Autodesk Inventor part; units mm, degrees
ref_plane "YZ Plane" through (0, 0, 0) normal (1, 0, 0) x (0, 1, 0)
ref_plane "XZ Plane" through (0, 0, 0) normal (0, 1, 0) x (-1, 0, 0)
ref_plane "XY Plane" through (0, 0, 0) normal (0, 0, 1) x (1, 0, 0)
sketch "スケッチ1" plane through (0, 0, 0) normal (0, 0, 1) x (1, 0, 0)
  line L0 (-75, -5) -> (-75, 5)
  line L1 (-75, 5) -> (10, 5)
  line L2 (10, 5) -> (10, -41.5)
  line L3 (10, -41.5) -> (0, -41.5)
  line L4 (0, -41.5) -> (0, -5)
  line L5 (0, -5) -> (-75, -5)
  point P0 (0, 0)
  dimension "d0" = 85
  dimension "d1" = 46.5
  dimension "d2" = 10
  dimension "d3" = 10
  dimension "d4" = 10
  dimension "d6" = 5
extrude "押し出し1" add sketch "スケッチ1" along normal blind 5 and the other way blind 5
sketch "スケッチ2" plane through (0, -41.5, 5) normal (0, -1, 0) x (1, 0, 0)
  circle A0 centre (5, -5) radius 7.5
  line L0 (0, -10) -> (0, 0)
  point P0 (0, -5)
  point P1 (0, -5)
  dimension "d11" = 15
  dimension "d12" = 5
  dimension "d13" = 5
extrude "押し出し2" add sketch "スケッチ2" against normal blind 20
sketch "スケッチ3" plane through (-75, -5, 5) normal (-1, 0, 0) x (0, 0, 1)
  circle A0 centre (-5, 5) radius 7.5
  dimension "d16" = 15
extrude "押し出し3" add sketch "スケッチ3" against normal blind 20
properties part number "r_link_wr2wp"
Could you check a few things on this model? Use its own coordinates, in mm. A direction names the side the tool comes from. Give positions to 0.01 mm unless a question says otherwise; leave off trailing zeros. Order: outer loops, then holes, each group sorted by start corner. A loop starts at its lowest first (then second) coordinate and runs counter-clockwise, first axis right, second up.
1. Suppose I cut it at A-A (z = 0). Write out the boundary of the cut face in (x, y), plus the area to 4 significant figures.
Answers below:
outline: (-75, -7.5) - (-55, -7.5) - (-55, -5) - (0, -5) - (0, -21.5) - (-2.5, -21.5) - (-2.5, -41.5) - (12.5, -41.5) - (12.5, -21.5) - (10, -21.5) - (10, 5) - (-55, 5) - (-55, 7.5) - (-75, 7.5) - close
area: 1,415 mm2
2. For pin 1 (4.5 mm diameter, centred on x = 2, z = 1.5, fed in from +Y); pin 2 (5 mm diameter, centred on y = -12, z = -1, fed in from -X); pin 3 (5 mm diameter, centred on x = -41, z = 0.5, fed in from -Y), each with a flat end and sliding along its axis, tell me the tip position at first contact or that it passes through.
Answers below:
pin 1: stops at y = 5
pin 2: stops at x = 0
pin 3: stops at y = -5
3. Suppose I cut it at B-B (x = 5). Write out the boundary of the cut face in (y, z), plus the area to 3 significant figures.
Answers below:
outline: (-41.5, -7.5) - (-21.5, -7.5) - (-21.5, -5) - (5, -5) - (5, 5) - (-21.5, 5) - (-21.5, 7.5) - (-41.5, 7.5) - close
area: 565 mm2
4. Thinking about a two-plate mould opening in X: for faces 4 (the flat face through (-55, 1, -6)), 5 (the cylindrical face through (-65.14, 0.33, -7.493)), 6 (the flat face through (10, -8, 0)), which applies, +X half, -X half, draft (parallel to the pull), parting line (faces both ways), or undercut?
Answers below:
face 4: undercut
face 5: draft
face 6: +X half
5. Which directions (+Z, -Z, +X, -X, +Y, -Y) give clear straight access to the entire face, cutting with the end or side of a thin tool? Please do faces 1 (the flat face through (-23, 5, 0)), 2 (the flat face through (-16, -2, -5)), 3 (the flat face through (-1, -21.5, 1)).
Answers below:
face 1: +Z, -Z, +X, +Y
face 2: -Z, +X, +Y
face 3: none
6. Suppose I cut it at D-D (x = -7). Write out the boundary of the cut face in (y, z).
Answers below:
outline: (-5, -5) - (5, -5) - (5, 5) - (-5, 5) - close
7. Suppose I cut it at C-C (y = 0). Write out the boundary of the cut face in (x, z).
Answers below:
outline: (-75, -7.5) - (-55, -7.5) - (-55, -5) - (10, -5) - (10, 5) - (-55, 5) - (-55, 7.5) - (-75, 7.5) - close
8. I need wall thicknesses on L1, parallel to X at y = -6.5, z = -1.75; L2, parallel to X at y = -13.5, z = 2; L3, parallel to Y at x = -16, z = -3.75. Which ranges of each line are inside material? Lowest first, please.
Answers below:
L1: x = -75 to -55, 0 to 10
L2: x = 0 to 10
L3: y = -5 to 5
